from build123d import *

# Parameters (mm, degrees)
BOSS_EXTRUDE2_DEPTH = 8
FILLET1_R           = 10
FILLET3_R           = 5
FILLET4_R           = 5
SKETCH3_R           = 5
BOSS_EXTRUDE3_DEPTH = 10
SKETCH2_R           = 5
BOSS_EXTRUDE4_DEPTH = 18
SKETCH4_R           = 4
BOSS_EXTRUDE5_DEPTH = 10
CUT_EXTRUDE1_START  = -8
CUT_EXTRUDE1_DEPTH  = 8
SKETCH7_W           = 0.7
SKETCH7_H           = 1.2
CIRPATTERN1_COUNT   = 3


with BuildPart() as part:
    # Sketch1 → Boss-Extrude2 (new body)
    with BuildSketch(Plane.YZ):
        with BuildLine():
            Line((-19.991801075, -0.572616617), (-46.319219382, -15.772758664))
            Line((-46.319219382, -15.772758664), (-36.819219382, -32.227241336))
            Line((-36.819219382, -32.227241336), (-10.491801075, -17.027099289))
            ThreePointArc((-10.491801075, -17.027099289), (0, -20), (10.491801075, -17.027099289))
            Line((10.491801075, -17.027099289), (36.819219382, -32.227241336))
            Line((36.819219382, -32.227241336), (46.319219382, -15.772758664))
            Line((46.319219382, -15.772758664), (19.991801075, -0.572616617))
            ThreePointArc((19.991801075, -0.572616617), (17.320508076, 10), (9.5, 17.599715907))
            Line((9.5, 17.599715907), (9.5, 48))
            Line((9.5, 48), (-9.5, 48))
            Line((-9.5, 48), (-9.5, 17.599715907))
            ThreePointArc((-9.5, 17.599715907), (-17.320508076, 10), (-19.991801075, -0.572616617))
        make_face()
    extrude(amount=BOSS_EXTRUDE2_DEPTH)

    # Fillet1
    fillet1_edges = [part.edges().sort_by_distance(p)[0] for p in [
        (4, 9.5, 17.599715907),
        (4, 19.991801075, -0.572616617),
        (4, 10.491801075, -17.027099289),
        (4, -10.491801075, -17.027099289),
        (4, -19.991801075, -0.572616617),
        (4, -9.5, 17.599715907),
    ]]
    fillet(fillet1_edges, radius=FILLET1_R)

    # Fillet3
    fillet3_edges = [part.edges().sort_by_distance(p)[0] for p in [
        (4, -9.5, 48),
        (4, 9.5, 48),
    ]]
    fillet(fillet3_edges, radius=FILLET3_R)

    # Fillet4
    fillet4_edges = [part.edges().sort_by_distance(p)[0] for p in [
        (4, 46.319219382, -15.772758664),
        (4, 36.819219382, -32.227241336),
        (4, -36.819219382, -32.227241336),
        (4, -46.319219382, -15.772758664),
    ]]
    fillet(fillet4_edges, radius=FILLET4_R)

    # Sketch3 → Boss-Extrude3 (add)
    with BuildSketch(Plane(origin=(0, 0, 0), x_dir=(0, -1, 0), z_dir=(-1, 0, 0))):
        with Locations(Location((0, 0, 0), (0, 0, 270))):
            Circle(SKETCH3_R)
    extrude(amount=BOSS_EXTRUDE3_DEPTH)

    # Sketch2 → Boss-Extrude4 (add)
    with BuildSketch(Plane(origin=(0, 0, 0), x_dir=(0, -1, 0), z_dir=(-1, 0, 0))):
        with Locations(Location((0, 42, 0), (0, 0, 270))):
            Circle(SKETCH2_R)
        with Locations(Location((-36.373066959, -21, 0), (0, 0, 270))):
            Circle(SKETCH2_R)
        with Locations(Location((36.373066959, -21, 0), (0, 0, 270))):
            Circle(SKETCH2_R)
    extrude(amount=BOSS_EXTRUDE4_DEPTH)

    # Sketch4 → Boss-Extrude5 (add)
    with BuildSketch(Plane.YZ.offset(8)):
        with Locations(Location((0, 0, 0), (0, 0, 270))):
            Circle(SKETCH4_R)
    extrude(amount=BOSS_EXTRUDE5_DEPTH)

    # Sketch5 → Cut-Extrude1 (cut)
    with BuildSketch(Plane.YZ.offset(18).offset(CUT_EXTRUDE1_START)):
        with BuildLine():
            Line((-3.2, -2.4), (3.2, -2.4))
            ThreePointArc((3.2, -2.4), (0, -4), (-3.2, -2.4))
        make_face()
    extrude(amount=CUT_EXTRUDE1_DEPTH, mode=Mode.SUBTRACT)

    # Sketch7 → Cut-Revolve1 (revolve, cut)
    with BuildSketch(Plane(origin=(0, 0, 0), x_dir=(-1, 0, 0), z_dir=(0, 1, 0))):
        with Locations((8.35, 47)):
            Rectangle(SKETCH7_W, SKETCH7_H)
        with Locations((17.05, 47)):
            Rectangle(SKETCH7_W, SKETCH7_H)
    cut_revolve1 = revolve(axis=Axis((-21.815535784, 0, 42), (1, 0, 0)), mode=Mode.SUBTRACT)

    # CirPattern1: Cut-Revolve1 ×3 about axis
    cirpattern1_axis = Axis((0, 0, 0), (1, 0, 0))
    for i in range(1, CIRPATTERN1_COUNT):
        add(cut_revolve1.rotate(cirpattern1_axis, i * 360 / CIRPATTERN1_COUNT), mode=Mode.SUBTRACT)


solid = part.part
Read the model definition and answer for the solid it produces. Units are mm, in the model's axes. A direction names the side the tool comes from. Coordinates: 2 decimals unless noted, no trailing zeros. Write each loop counter-clockwise with the first axis right and the second up, starting at its lowest first coordinate (ties: lowest second). Pieces come first, ordered by that corner, then holes. Notation, with made-up numbers: (68.5, 79) - (81.5, 79) arc R18 ccw to (81.5, 89) - close; hole circle Ø3 at (-17, -9.75). An arc over 180 degrees is marked (long way). One line per question, with ' | ' between items.
Q1. Find section C-C, the plane x = 7. Write down the section's boundary in (y, z), plus the area to 3 significant figures.
Result set:
outline: (-43.82, -20.1) - (-39.32, -27.9) arc R5 ccw to (-32.49, -29.73) - (-14.99, -19.63) arc R10 cw to (-6.66, -18.86) arc R20 ccw to (6.66, -18.86) arc R10 cw to (14.99, -19.63) - (32.49, -29.73) arc R5 ccw to (39.32, -27.9) - (43.82, -20.1) arc R5 ccw to (41.99, -13.27) - (24.49, -3.17) arc R10 cw to (19.66, 3.66) arc R20 ccw to (13, 15.2) arc R10 cw to (9.5, 22.8) - (9.5, 43) arc R5 ccw to (4.5, 48) - (-4.5, 48) arc R5 ccw to (-9.5, 43) - (-9.5, 22.8) arc R10 cw to (-13, 15.2) arc R20 ccw to (-19.66, 3.66) arc R10 cw to (-24.49, -3.17) - (-41.99, -13.27) arc R5 ccw to start | area: 2,890 mm^2
Q2. Find section B-B, the plane z = 42. Write down the section's boundary in (x, y).
Result set:
outline: (-18, -5) - (-17.4, -5) - (-17.4, -4.4) - (-16.7, -4.4) - (-16.7, -5) - (-8.7, -5) - (-8.7, -4.4) - (-8, -4.4) - (-8, -5) - (0, -5) - (0, -9.5) - (8, -9.5) - (8, 9.5) - (0, 9.5) - (0, 5) - (-8, 5) - (-8, 4.4) - (-8.7, 4.4) - (-8.7, 5) - (-16.7, 5) - (-16.7, 4.4) - (-17.4, 4.4) - (-17.4, 5) - (-18, 5) - close
Q3. Consider L1, parallel to Y at x = 6, z = 28; L2, parallel to X at y = -25, z = -21.5; L3, parallel to Y at x = -6.5, z = -21.5. Determine where each line is inside the solid, lowest interval first. Write a range as [from, to].
Result set:
L1: [-9.5, 9.5] | L2: [0, 8] | L3: [-41.35, -31.4], [31.4, 41.35]
Q4. Find section D-D, the plane x = -6. Write down the section's boundary in (y, z).
Result set:
outline: circle Ø10 at (-36.37, -21); circle Ø10 at (0, 0); circle Ø10 at (0, 42); circle Ø10 at (36.37, -21)
Q5. For faces 1 (the flat face through (-17.4, 34, -25)), 2 (the flat face through (-10, 0, 0)), 3 (the cylindrical face through (-12.644, 41.254, -19.916)), determine the directions among +Z, -Z, +X, -X, +Y, -Y from which every point of the face is accessible in a straight line to the end or side of a thin tool.
Result set:
face 1: none | face 2: -Z, -X, +Y, -Y | face 3: -X
Q6. Determine the mould class of faces 4 (the flat face through (-8, 34, -25)), 5 (the flat face through (0, -1, -8)), 6 (the cylindrical face through (4.06, 8, 46.57)) for opening direction X: +X half, -X half, draft (parallel to the pull), parting line (faces both ways), or undercut.
Result set:
face 4: undercut | face 5: -X half | face 6: draft
Q7. Each of these flat-tipped pins is pushed along its axis until it touches: P1, Ø8, axis at y = -1.5, z = 41.5, coming from the +X side; P2, Ø4, axis at x = 3.5, z = 16, coming from the -Y side; P3, Ø12, axis at x = 1.5, z = -3, coming from the -Y side. Where does it stop, or does it pass through?
Result set:
P1: x = 8 | P2: y = -14.28 | P3: y = -34.59
